Here's how the part is built. I have some questions about the finished solid (model axes, mm). A direction names the side the tool comes from. Round coordinates to 2 decimals unless told otherwise and drop trailing zeros. Order: outer loops, then holes, each group sorted by start corner. A loop starts at its lowest first (then second) coordinate and runs counter-clockwise, first axis right, second up. Notation, with made-up numbers: M -38,82.25 L -13,82.25 A33 cw -13,120.25 Z; hole C 79,11 d4. An arc over 180 degrees is marked long. Use one line per item in the form item = value. Start each with the question number.
```python
from build123d import *

# Parameters (mm, degrees)
BOTTOM_HORIZONTAL_ANGLE_DEPTH   = 1574.8
BOTTOM_HORIZONTAL_ANGLE_2_DEPTH = 1574.8
FRONT_VERTIAL_ANGLE_DEPTH       = 406.4
REAR_VERTICAL_ANGLE_DEPTH       = 609.6
REAR_TOP_HORIZONTAL_ANGLE_DEPTH = 609.6
BOSS_EXTRUDE5_DEPTH             = 986.357582
BOSS_EXTRUDE6_REACH             = 1011.65


with BuildPart() as part:
    # Sketch5 → Bottom Horizontal Angle (new body)
    with BuildSketch(Plane(origin=(0, 0, 0), x_dir=(0, 0, -1), z_dir=(1, 0, 0))):
        Polygon((-504.825, -304.8), (-504.825, -254), (-501.65, -254), (-501.65, -301.625), (-454.025, -301.625), (-454.025, -304.8), align=None)
    extrude(amount=BOTTOM_HORIZONTAL_ANGLE_DEPTH)



with BuildPart() as body_2:
    # Sketch5 → Bottom Horizontal Angle 2 (new body)
    with BuildSketch(Plane(origin=(0, 0, 0), x_dir=(0, 0, -1), z_dir=(1, 0, 0))):
        Polygon((501.65, -254), (504.825, -254), (504.825, -304.8), (454.025, -304.8), (454.025, -301.625), (501.65, -301.625), align=None)
    extrude(amount=BOTTOM_HORIZONTAL_ANGLE_2_DEPTH)


with BuildPart() as part_1:
    add(part.part)

    add(body_2.part)  # Front Vertial Angle merges body 2
    # Sketch6 → Front Vertial Angle (add)
    with BuildSketch(Plane.XZ.offset(304.8)):
        Polygon((1574.8, -504.825), (1524, -504.825), (1524, -501.65), (1571.625, -501.65), (1571.625, -454.025), (1574.8, -454.025), align=None)
        Polygon((1524, 501.65), (1524, 504.825), (1574.8, 504.825), (1574.8, 454.025), (1571.625, 454.025), (1571.625, 501.65), align=None)
    extrude(amount=-FRONT_VERTIAL_ANGLE_DEPTH)

    # Sketch7 → Rear Vertical Angle (add)
    with BuildSketch(Plane.XZ.offset(304.8)):
        Polygon((0, 504.825), (50.8, 504.825), (50.8, 501.65), (3.175, 501.65), (3.175, 454.025), (0, 454.025), align=None)
        Polygon((50.8, -501.65), (50.8, -504.825), (0, -504.825), (0, -454.025), (3.175, -454.025), (3.175, -501.65), align=None)
    extrude(amount=-REAR_VERTICAL_ANGLE_DEPTH)

    # Sketch8 → Rear Top Horizontal Angle (add)
    with BuildSketch(Plane.ZY):
        Polygon((504.825, 304.8), (504.825, 254), (501.65, 254), (501.65, 301.625), (454.025, 301.625), (454.025, 304.8), align=None)
        Polygon((-501.65, 254), (-504.825, 254), (-504.825, 304.8), (-454.025, 304.8), (-454.025, 301.625), (-501.65, 301.625), align=None)
    extrude(amount=-REAR_TOP_HORIZONTAL_ANGLE_DEPTH)

    # Sketch10 → Boss-Extrude5 (add)
    with BuildSketch(Plane(origin=(522.283289125, -109.954376658, 0), x_dir=(0, 0, -1), z_dir=(0.978549785, -0.206010481, 0))):
        Polygon((504.825, 423.845963712), (504.825, 373.045963712), (501.65, 373.045963712), (501.65, 420.670963712), (454.025, 420.670963712), (454.025, 423.845963712), align=None)
        Polygon((-501.65, 373.045963712), (-504.825, 373.045963712), (-504.825, 423.845963712), (-454.025, 423.845963712), (-454.025, 420.670963712), (-501.65, 420.670963712), align=None)
    extrude(amount=BOSS_EXTRUDE5_DEPTH)

    # Sketch11 → Boss-Extrude6 (add, up to next)
    with BuildSketch(Plane(origin=(0, 0, -504.825), x_dir=(-1, 0, 0), z_dir=(0, 0, -1)), mode=Mode.PRIVATE) as boss_extrude6_sk1:
        Polygon((-1574.8, 101.6), (-1524, 101.6), (-1524, 98.425), (-1571.625, 98.425), (-1571.625, 50.8), (-1574.8, 50.8), align=None)
    boss_extrude6_tool1 = extrude(boss_extrude6_sk1.sketch, amount=-BOSS_EXTRUDE6_REACH, mode=Mode.PRIVATE) - part_1.part
    add(boss_extrude6_tool1.solids().sort_by_distance((1549.4, 100.88158, -504.825))[0])
    # Sketch11 → Boss-Extrude6 (add, up to next)
    with BuildSketch(Plane(origin=(0, 0, -504.825), x_dir=(-1, 0, 0), z_dir=(0, 0, -1)), mode=Mode.PRIVATE) as boss_extrude6_sk2:
        Polygon((-1524, -301.625), (-1524, -304.8), (-1574.8, -304.8), (-1574.8, -254), (-1571.625, -254), (-1571.625, -301.625), align=None)
    boss_extrude6_tool2 = extrude(boss_extrude6_sk2.sketch, amount=-BOSS_EXTRUDE6_REACH, mode=Mode.PRIVATE) - part_1.part
    add(boss_extrude6_tool2.solids().sort_by_distance((1524.71842, -303.2125, -504.825))[0])
    # Sketch11 → Boss-Extrude6 (add, up to next)
    with BuildSketch(Plane(origin=(0, 0, -504.825), x_dir=(-1, 0, 0), z_dir=(0, 0, -1)), mode=Mode.PRIVATE) as boss_extrude6_sk3:
        Polygon((0, -304.8), (-50.8, -304.8), (-50.8, -301.625), (-3.175, -301.625), (-3.175, -254), (0, -254), align=None)
    boss_extrude6_tool3 = extrude(boss_extrude6_sk3.sketch, amount=-BOSS_EXTRUDE6_REACH, mode=Mode.PRIVATE) - part_1.part
    add(boss_extrude6_tool3.solids().sort_by_distance((25.4, -304.08158, -504.825))[0])
    # Sketch11 → Boss-Extrude6 (add, up to next)
    with BuildSketch(Plane(origin=(0, 0, -504.825), x_dir=(-1, 0, 0), z_dir=(0, 0, -1)), mode=Mode.PRIVATE) as boss_extrude6_sk4:
        Polygon((-3.175, 301.625), (-50.8, 301.625), (-50.8, 304.8), (0, 304.8), (0, 254), (-3.175, 254), align=None)
    boss_extrude6_tool4 = extrude(boss_extrude6_sk4.sketch, amount=-BOSS_EXTRUDE6_REACH, mode=Mode.PRIVATE) - part_1.part
    add(boss_extrude6_tool4.solids().sort_by_distance((26.9875, 302.34342, -504.825))[0])
    # Sketch11 → Boss-Extrude6 (add, up to next)
    with BuildSketch(Plane(origin=(0, 0, -504.825), x_dir=(-1, 0, 0), z_dir=(0, 0, -1)), mode=Mode.PRIVATE) as boss_extrude6_sk5:
        Polygon((-605.340190101, 263.281530829), (-644.735373854, 295.354252838), (-642.730828729, 297.816451822), (-605.79784396, 267.748274939), (-575.729667077, 304.681259707), (-573.267468092, 302.676714582), align=None)
    boss_extrude6_tool5 = extrude(boss_extrude6_sk5.sketch, amount=-BOSS_EXTRUDE6_REACH, mode=Mode.PRIVATE) - part_1.part
    add(boss_extrude6_tool5.solids().sort_by_distance((624.516329, 279.958397, -504.825))[0])


solid = part_1.part
```
1) If I drill on line 1 (X direction, y = -275, z = -271) (3 decimals); line 2 (Z direction, x = 884, y = -275.5) (3 decimals); line 3 (X direction, y = 76.5, z = -403.5) (3 decimals), over which ranges is the centre line in solid material (lowest first)?
2) If we section it at A-A on y = -233.5: Write out the boundary of the cut face in (x, z) (3 decimals), then the cut area to 3 significant figures.
3) On a 3-axis mill with a long thin cutter (end or side, diameter ignored), from which of +Z, -Z, +X, -X, +Y, -Y can I reach the whole of each face in a straight line? I mean faces 1 (the flat face through (849, -301.625, 481)), 2 (the flat face through (1057.717, 158.546, 503.215)), 3 (the flat face through (1085.444, 204.622, -479.069)). Say none if no direction works.
4) Will these pins go through, and if not, where does the flat tip stop? pin 1 Ø5 at (x, z) = (593, -53.5) entering from +Y; pin 2 Ø3.5 at (x, z) = (1573, 131.5) entering from +Y.
5) If we section it at C-C on z = -210.5: Give the number of separate pieces and of enclosed holes in the cut face, then the cut area to 3 significant figures.
6) If we section it at B-B on x = 308: Write out the boundary of the cut face in (y, z) (3 decimals), then the cut area to 3 significant figures.
7) If we mould it in two halves opening along Y, with no side actions, what happens to faces 4 (the flat face through (1085.444, 204.622, 479.781)), 5 (the flat face through (1574.8, -268, -40)), 6 (the flat face through (1571.625, 62, -40))? For each: +Y half, -Y half, draft (parallel to the pull), parting line (faces both ways), or undercut.
Completed:
q1.line_1 = 0 to 3.175, 1571.625 to 1574.8
q1.line_2 = -504.825 to -501.65, 501.65 to 504.825
q1.line_3 = 1571.625 to 1574.8
q2.outline = M 0,-504.825 L 50.8,-504.825 L 50.8,-501.65 L 3.175,-501.65 L 3.175,-454.025 L 0,-454.025 Z; M 0,454.025 L 3.175,454.025 L 3.175,501.65 L 50.8,501.65 L 50.8,504.825 L 0,504.825 Z; M 1524,-504.825 L 1574.8,-504.825 L 1574.8,-454.025 L 1571.625,-454.025 L 1571.625,-501.65 L 1524,-501.65 Z; M 1524,501.65 L 1571.625,501.65 L 1571.625,454.025 L 1574.8,454.025 L 1574.8,504.825 L 1524,504.825 Z
q2.area = 1,250 mm²
q3.face_1 = none
q3.face_2 = +Z, -Z
q3.face_3 = +Z, -Z, +X, +Y
q4.pin_1 = 286.54
q4.pin_2 = 101.6
q5.separate_pieces = 5
q5.enclosed_holes = 0
q5.area = 1,560 mm²
q6.outline = M -304.8,-504.825 L -254,-504.825 L -254,-501.65 L -301.625,-501.65 L -301.625,-454.025 L -304.8,-454.025 Z; M -304.8,454.025 L -301.625,454.025 L -301.625,501.65 L -254,501.65 L -254,504.825 L -304.8,504.825 Z; M 254,-504.825 L 304.8,-504.825 L 304.8,-454.025 L 301.625,-454.025 L 301.625,-501.65 L 254,-501.65 Z; M 254,501.65 L 301.625,501.65 L 301.625,454.025 L 304.8,454.025 L 304.8,504.825 L 254,504.825 Z
q6.area = 1,250 mm²
q7.face_4 = +Y half
q7.face_5 = draft
q7.face_6 = undercut
